For this review, take the finished solid that the model builds, in its own axes (mm). Face numbers are marked on the shaded views. A direction names the side the tool comes from. Round coordinates to 2 decimals unless told otherwise and drop trailing zeros. Order: outer loops, then holes, each group sorted by start corner. A loop starts at its lowest first (then second) coordinate and runs counter-clockwise, first axis right, second up. Notation, with made-up numbers: M 25,75 L 45,75 A21 ccw 45,98 Z; hole C 22.5,21 d8. An arc over 180 degrees is marked long. Put each result on its own line as item: value.
from build123d import *


with BuildPart() as f2:
    # F2: sweep along a path in F1
    with BuildLine(Plane.YZ) as f2_path:
        Line((0, 0), (-8.0247949809, 24.9660369009))
    # F0 (on Top) → F2 (sweep)
    with BuildSketch(Plane.XY):
        Polygon((-0.1032873551, 21.0342315395), (-20.0366605189, 6.4017028972), (-12.2800498667, -17.0777615631), (12.4471723178, -16.956339995), (19.9728254229, 6.5981671214), align=None)
    sweep(path=f2_path.line)

    # F3: sweep along a path in F1
    with BuildLine(Plane.YZ) as f3_path:
        Line((-8.0247949809, 24.9660369009), (22.6477645338, 61.3451190293))
    # F2_face (on face) → F3 (sweep)
    with BuildSketch(Plane(origin=(0, -8.0247949809, 24.9660369009), x_dir=(1, 0, 0), z_dir=(0, 0, 1))):
        Polygon((12.4471723178, -16.956339995), (19.9728254229, 6.5981671214), (-0.1032873551, 21.0342315395), (-20.0366605189, 6.4017028972), (-12.2800498667, -17.0777615631), align=None)
    sweep(path=f3_path.line)

    # F2_face1 (on face) → F4 section 0
    with BuildSketch(Plane(origin=(0, 0, 0), x_dir=(1, 0, 0), z_dir=(0, 0, -1)), mode=Mode.PRIVATE) as f4_s0:
        Polygon((19.9728254229, -6.5981671214), (12.4471723178, 16.956339995), (-12.2800498667, 17.0777615631), (-20.0366605189, -6.4017028972), (-0.1032873551, -21.0342315395), align=None)
    loft([f4_s0.sketch, Vertex(0, 22.2911071032, -57.4218854308)])


solid = f2.part
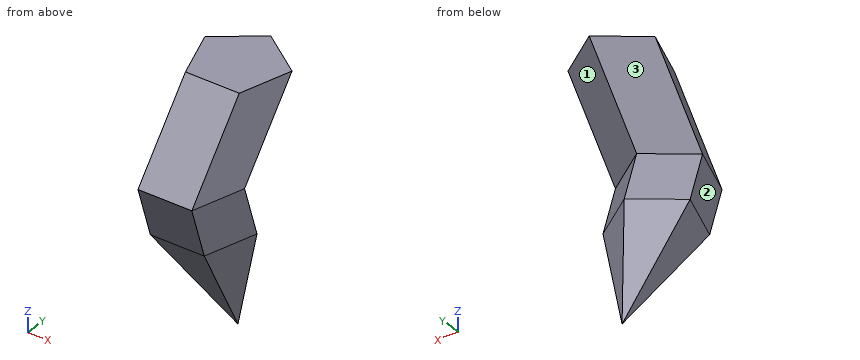
(1) Add section B-B on x = 2. Give the boundary of the cut face in (y, z).
A:
outline: M -25.03,24.97 L -17.01,0 L 15.98,-48.2 L 20.72,-51.67 L 19.52,0 L 11.5,24.97 L 42.17,61.35 L 5.64,61.35 Z
(2) Insertion check: pin 1 Ø10 at (x, z) = (-13, 6.5) entering from +Y; pin 2 Ø1 at (x, y) = (14, 12.5) entering from -Z; pin 3 Ø6 at (x, y) = (8, -2.5) entering from -Z. Each pin has a flat end and moves straight along its axis. Give the tip position at first contact, or say it passes through.
A:
pin 1: stops at y = 13.48
pin 2: stops at z = 35.66
pin 3: stops at z = -25.27
(3) Add section C-C on z = 40.5. Give the boundary of the cut face in (x, y).
A:
outline: M -20.04,11.47 L -12.28,-12.01 L 12.45,-11.88 L 19.97,11.67 L -0.1,26.11 Z
(4) For the marked faces 1, 2 and 3, list the 3-axis set-ups (+Z, -Z, +X, -X, +Y, -Y) from which the entire face can be reached by the end or side of a thin tool; tool diameter is ignored.
A:
face 1: +X, +Y
face 2: -Z, -X, -Y
face 3: -X, +Y
(5) Add section D-D on y = -7.5. Give the boundary of the cut face in (x, z).
A:
outline: M -18.1,24.97 L -15.44,0 L -9.29,-13.97 L 9.45,-13.84 L 15.47,0 L 18.03,24.97 L 12.45,45.7 L -12.28,45.84 Z
(6) To check wall thickness, follow L1, parallel to Z at x = -12, y = 21.5; L2, parallel to Z at x = 11.5, y = 27; L3, parallel to X at y = -5, z = 13. State the ranges of each line that lie inside material, in increasing order.
A:
L1: z = 45.39 to 61.35
L2: z = 51.46 to 61.35
L3: x = -17.65 to 17.6
(7) Add section A-A on y = 15. Give the boundary of the cut face in (x, z).
A:
outline: M -20.04,44.68 L -0.1,27.33 L 19.97,44.45 L 15.42,61.35 L -15.4,61.35 Z; M -9.19,-31.07 L -2.27,-46.79 L 2.31,-46.75 L 9.28,-30.74 L 8.29,0 L -0.1,18.77 L -8.32,0 Z
